Read the model definition and answer for the solid it produces. Units are mm, in the model's axes. A direction names the side the tool comes from. Coordinates: 2 decimals unless noted, no trailing zeros. Loops run counter-clockwise (first coordinate to the right, second up) from the corner with the lowest first, then second, coordinate; pieces in that order, holes last. Notation, with made-up numbers: M 70,-11 L 99,-11 A22 ccw 99,-2 Z; hole C 32.5,22.25 d6. An arc over 180 degrees is marked long. One line per item, written item: value. Start each with the question number.
1. Flat-ended cylindrical pins translate along their axes: pin 1 (2 mm diameter, centred on x = 74.5, y = 37.5, fed in from +Z); pin 2 (1.1 mm diameter, centred on y = 29, z = -25, fed in from -X); pin 3 (3 mm diameter, centred on x = -73.5, z = -23, fed in from +Y); pin 4 (2.5 mm diameter, centred on x = 25, y = 28.5, fed in from +Z). Find the tip coordinate at first contact, or state that the pin passes through.
2. For faces 1 (the face through (-73.102, 25.493, -45.22)), 2 (the face through (18, 30, -24)), 3 (the face through (-74, -28, -23)), 4 (the face through (-72, -30, -24)), 5 (the face through (72, -35.5, -57)), determine the directions among +Z, -Z, +X, -X, +Y, -Y from which every point of the face is accessible in a straight line to the end or side of a thin tool.
3. The part is cut by section C-C (x = 7.5). Write down the section's boundary in (y, z).
4. The part is cut by section B-B (z = -34.5). State how many separate pieces and enclosed holes the cut face has, then the cut area to 3 significant figures.
5. Consider probe 1 along Y at (x, z) = (25, -46); probe 2 along Y at (x, z) = (43, -39); probe 3 along Y at (x, z) = (-65, -50). Determine where each line is inside the solid, lowest interval first.
6. Determine the mould class of faces 6 (the face through (-58.032, -27.972, -45.22)), 7 (the face through (72, 35.5, -57)), 8 (the face through (73, -38, -62.5)) for opening direction Y: +Y half, -Y half, draft (parallel to the pull), parting line (faces both ways), or undercut.
7. The part is cut by section A-A (x = 52). Write down the section's boundary in (y, z), then the cut area to 3 significant figures.
```python
from build123d import *

# Parameters (mm, degrees)
EXTRUDE136072_DEPTH                     = 12
CHAMFER002_SIZE                         = 1
EXTRUDE136071_DEPTH                     = 15
CHAMFER001_SIZE                         = 2
SKETCH295_R                             = 1.4
EXTRUDE136074_DEPTH                     = 50
EXTRUDE136076_DEPTH                     = 4
EXTRUDE136076_ONTO_SKETCH296_ROLL_ANGLE = 90
EXTRUDE136075_DEPTH                     = 4
EXTRUDE136075_ONTO_SKETCH296_ROLL_ANGLE = 90
BOX022_W                                = 25
BOX022_H                                = 80
BOX022_DEPTH                            = 51
EXTRUDE136056_DEPTH                     = 40
EXTRUDE136055_DEPTH                     = 42
FILLET_R                                = 2


with BuildPart() as chamfer002:
    # Sketch293 → Extrude136072 (new body)
    with BuildSketch(Plane.XY):
        Polygon((0, 37.5), (5, 37.5), (5, 35.5), (2, 35.5), align=None)
        Polygon((0, -37.5), (5, -37.5), (5, -35.5), (2, -35.5), align=None)
    extrude(amount=-EXTRUDE136072_DEPTH)


with BuildPart() as chamfer002_1:
    # Extrude136072 placement: moved
    add(chamfer002.part.moved(Location((4, 0, 6))))

    # Chamfer002
    chamfer002_edges = [chamfer002_1.edges().sort_by_distance(p)[0] for p in [
        (7.5, -35.5, 6),
        (7.5, 35.5, 6),
    ]]
    chamfer(chamfer002_edges, length=CHAMFER002_SIZE)


with BuildPart() as fusion034004041070:
    # Sketch292 → Extrude136071 (new body)
    with BuildSketch(Plane.YZ):
        Polygon((-40, 8.5), (-37.5, 6), (-37.5, -6), (-40, -6), align=None)
        Polygon((40, 8.5), (37.5, 6), (37.5, -6), (40, -6), align=None)
    extrude(amount=EXTRUDE136071_DEPTH)

    # Chamfer001
    chamfer001_edges = [fusion034004041070.edges().sort_by_distance(p)[0] for p in [
        (0, 37.5, 0),
        (0, -37.5, 0),
    ]]
    chamfer(chamfer001_edges, length=CHAMFER001_SIZE)


with BuildPart() as fusion034004041070_1:
    # Chamfer001 placement: moved
    add(fusion034004041070.part.moved(Location((1.5, 0, 0))))

    # Fusion034004041070: union Chamfer002
    add(chamfer002_1.part)


with BuildPart() as fusion034004041070_2:
    # Fusion034004041070 placement: moved
    add(fusion034004041070_1.part.moved(Location((64.5, 0, -31))))


with BuildPart() as fusion034004041071:
    # Sketch295 → Extrude136074 (new body)
    with BuildSketch(Plane.XY):
        with Locations((-65, 28.5)):
            Circle(SKETCH295_R)
        with Locations((25, 28.5)):
            Circle(SKETCH295_R)
        with Locations((-65, -28.5)):
            Circle(SKETCH295_R)
        with Locations((25, -28.5)):
            Circle(SKETCH295_R)
    extrude(amount=-EXTRUDE136074_DEPTH)

    # Fusion034004041071: union Fusion034004041070
    add(fusion034004041070_2.part)


with BuildPart() as extrude136076:
    # Sketch296 as drawn → Extrude136076 (new)
    with BuildSketch(Plane.XY):
        Polygon((-77, 3.5), (-72, 3.5), (-72, 0), (-75, 0), (-75, 1), (-77, 3), align=None)
        Polygon((15, 0), (15, 1), (13, 3), (13, 3.5), (18, 3.5), (18, 0), align=None)
    extrude(amount=-EXTRUDE136076_DEPTH)


with BuildPart() as extrude136076_1:
    # Extrude136076 onto Sketch296 roll: moved
    add(extrude136076.part.rotate(Axis((0, 0, 0), (1, 0, 0)), EXTRUDE136076_ONTO_SKETCH296_ROLL_ANGLE))


with BuildPart() as extrude136076_2:
    # Extrude136076 onto Sketch296 placement: moved
    add(extrude136076_1.part.moved(Location((0, -2, 0))))


with BuildPart() as extrude136076_3:
    # Extrude136076 placement: moved
    add(extrude136076_2.part.moved(Location((0, -30, 0))))


with BuildPart() as fusion034004041067:
    # Sketch296 as drawn → Extrude136075 (new)
    with BuildSketch(Plane.XY):
        Polygon((-77, 3.5), (-72, 3.5), (-72, 0), (-75, 0), (-75, 1), (-77, 3), align=None)
        Polygon((15, 0), (15, 1), (13, 3), (13, 3.5), (18, 3.5), (18, 0), align=None)
    extrude(amount=-EXTRUDE136075_DEPTH)


with BuildPart() as fusion034004041067_1:
    # Extrude136075 onto Sketch296 roll: moved
    add(fusion034004041067.part.rotate(Axis((0, 0, 0), (1, 0, 0)), EXTRUDE136075_ONTO_SKETCH296_ROLL_ANGLE))


with BuildPart() as fusion034004041067_2:
    # Extrude136075 onto Sketch296 placement: moved
    add(fusion034004041067_1.part.moved(Location((0, -2, 0))))


with BuildPart() as fusion034004041067_3:
    # Extrude136075 placement: moved
    add(fusion034004041067_2.part.moved(Location((0, 30, 0))))

    # Fusion034004041067: union Extrude136076
    add(extrude136076_3.part)


with BuildPart() as cube019:
    # Box022 → Box022 (new body)
    with BuildSketch(Plane(origin=(80, -40, -44), x_dir=(1, 0, 0), z_dir=(0, 0, 1))):
        with Locations((12.5, 40)):
            Rectangle(BOX022_W, BOX022_H)
    extrude(amount=BOX022_DEPTH)


with BuildPart() as extrude136056:
    # Sketch277 → Extrude136056 (new body)
    with BuildSketch(Plane.XY):
        with BuildLine():
            ThreePointArc((81.0383, -34.5), (85.059706, 0), (81.0383, 34.5))
            Line((66.5383, 34.5), (81.0383, 34.5))
            Line((63.0383, 38), (66.5383, 34.5))
            Line((40.0383, 38), (63.0383, 38))
            Line((27.5383, 25.5), (40.0383, 38))
            Line((12.636376, 25.5), (27.5383, 25.5))
            Line((10.0383, 30), (12.636376, 25.5))
            Line((10.0383, 30), (-52.9617, 30))
            Line((-62.9617, 26), (-52.9617, 30))
            Line((-82.9617, 25), (-62.9617, 26))
            ThreePointArc((-82.9617, 25), (-85.059706, 0), (-82.9617, -25))
            Line((-82.9617, -25), (-62.9617, -26))
            Line((-62.9617, -26), (-52.9617, -30))
            Line((10.0383, -30), (-52.9617, -30))
            Line((10.0383, -30), (12.636376, -25.5))
            Line((12.636376, -25.5), (27.5383, -25.5))
            Line((27.5383, -25.5), (40.0383, -38))
            Line((40.0383, -38), (63.0383, -38))
            Line((63.0383, -38), (66.5383, -34.5))
            Line((66.5383, -34.5), (81.0383, -34.5))
        make_face()
    extrude(amount=-EXTRUDE136056_DEPTH)


with BuildPart() as batteryboxfillet:
    # Sketch276 → Extrude136055 (new body)
    with BuildSketch(Plane.XY):
        with BuildLine():
            ThreePointArc((-84.489299, 32), (-87.942378, 0), (-84.489299, -32))
            Line((-84.489299, -32), (29.510701, -32))
            Line((29.510701, -32), (37.510701, -40))
            Line((37.510701, -40), (82.510701, -40))
            ThreePointArc((82.510701, -40), (87.942378, 0), (82.510701, 40))
            Line((37.510701, 40), (82.510701, 40))
            Line((29.510701, 32), (37.510701, 40))
            Line((-84.489299, 32), (29.510701, 32))
        make_face()
    extrude(amount=-EXTRUDE136055_DEPTH)

    # Cut009010006006006005016: cut Extrude136056
    add(extrude136056.part, mode=Mode.SUBTRACT)

    # Cut009010006006006005021: cut Cube019
    add(cube019.part, mode=Mode.SUBTRACT)

    # Fusion034004041068: union Fusion034004041067
    add(fusion034004041067_3.part)

    # Cut009010006006006005024: cut Fusion034004041071
    add(fusion034004041071.part, mode=Mode.SUBTRACT)

    # Fillet
    fillet_edges = [batteryboxfillet.edges().sort_by_distance(p)[0] for p in [
        (-84.489299, 32, -21),
        (-84.489299, -32, -21),
        (-87.942378, 0, -42),
        (-27.489299, 32, -42),
        (-27.489299, -32, -42),
        (33.510701, 36, -42),
        (58.755351, 40, -42),
        (33.510701, -36, -42),
        (58.755351, -40, -42),
        (37.510701, 40, -21),
        (37.510701, -40, -21),
    ]]
    fillet(fillet_edges, radius=FILLET_R)


with BuildPart() as batteryboxfillet_1:
    # Fillet placement: moved
    add(batteryboxfillet.part.moved(Location((0, 0, -25.5))))


solid = batteryboxfillet_1.part
```
Answer block:
1. pin 1: stops at z = -25.5
1. pin 2: stops at x = -85.16
1. pin 3: stops at y = 32
1. pin 4: passes through
2. face 1: +Z
2. face 2: +Z, +X, +Y, -Y
2. face 3: +Z, +X, -X
2. face 4: +Z, +Y, -Y
2. face 5: -Y
3. outline: M -32,-65.5 A2 ccw -30,-67.5 L 30,-67.5 A2 ccw 32,-65.5 L 32,-25.5 L 30,-25.5 L 30,-65.5 L -30,-65.5 L -30,-25.5 L -32,-25.5 Z
4. separate pieces: 1
4. enclosed holes: 4
4. area: 1,330 mm2
5. probe 1: y = -32 to -29.9, -27.1 to -25.5, 25.5 to 27.1, 29.9 to 32
5. probe 2: y = -40 to -38, 38 to 40
5. probe 3: y = -32 to -29.9, -27.1 to -25.9, 25.9 to 27.1, 29.9 to 32
6. face 6: undercut
6. face 7: +Y half
6. face 8: draft
7. outline: M -40,-65.5 A2 ccw -38,-67.5 L 38,-67.5 A2 ccw 40,-65.5 L 40,-25.5 L 38,-25.5 L 38,-65.5 L -38,-65.5 L -38,-25.5 L -40,-25.5 Z
7. area: 318 mm2
